Input: part model. Units: mm. Frame: model coordinates. A direction names the side the tool comes from. Coordinates: 2 decimals unless noted, no trailing zeros. Loops run counter-clockwise (first coordinate to the right, second up) from the corner with the lowest first, then second, coordinate; pieces in that order, holes last. Notation, with made-up numbers: (81, 26.25) - (93, 26.25) arc R18 cw to (93, 59.25) - close; hole circle Ø7 at (2, 59). An arc over 180 degrees is marked (long way). Use one line per item in the form item = value.
from build123d import *

# Parameters (mm, degrees)
F0_R     = 4.7
F0_R_2   = 1.5
F1_DEPTH = 7


with BuildPart() as f1:
    # F0 (on Top) → F1 (new body)
    with BuildSketch(Plane.XY):
        with BuildLine():
            Line((-26.979165, -28.984375), (-19.81169, -30.632258))
            ThreePointArc((-19.81169, -30.632258), (-8.174057, -35.553103), (4.444148, -36.208947))
            Line((4.444148, -36.208947), (11.611623, -37.85683))
            Line((11.611623, -37.85683), (16.622468, -32.473556))
            ThreePointArc((16.622468, -32.473556), (25.136294, -26.438703), (31.593175, -18.240328))
            ThreePointArc((31.593175, -18.240328), (32.647405, -16.278367), (33.579942, -14.255729))
            Line((33.579942, -14.255729), (38.590788, -8.872455))
            Line((38.590788, -8.872455), (36.434159, -1.841298))
            ThreePointArc((36.434159, -1.841298), (34.876919, 10.69761), (29.135794, 21.953219))
            Line((29.135794, 21.953219), (26.979165, 28.984375))
            Line((26.979165, 28.984375), (19.81169, 30.632258))
            ThreePointArc((19.81169, 30.632258), (10.328442, 34.988021), (0, 36.480657))
            ThreePointArc((0, 36.480657), (-2.226223, 36.412666), (-4.444148, 36.208947))
            Line((-4.444148, 36.208947), (-11.611623, 37.85683))
            Line((-11.611623, 37.85683), (-16.622468, 32.473556))
            ThreePointArc((-16.622468, 32.473556), (-26.702862, 24.855492), (-33.579942, 14.255729))
            Line((-33.579942, 14.255729), (-38.590788, 8.872455))
            Line((-38.590788, 8.872455), (-36.434159, 1.841298))
            ThreePointArc((-36.434159, 1.841298), (-35.464736, -8.549317), (-31.593175, -18.240328))
            ThreePointArc((-31.593175, -18.240328), (-30.421182, -20.134299), (-29.135794, -21.953219))
            Line((-29.135794, -21.953219), (-26.979165, -28.984375))
        make_face()
        with Locations((-14.546111, -25.194604)):
            Circle(F0_R, mode=Mode.SUBTRACT)
        with Locations((-25.194604, -14.546111)):
            Circle(F0_R, mode=Mode.SUBTRACT)
        with Locations((-29.092222, 0)):
            Circle(F0_R, mode=Mode.SUBTRACT)
        with Locations((-9.353936, -15.969821)):
            Circle(F0_R_2, mode=Mode.SUBTRACT)
        with BuildLine():
            Line((-6.784947, -19.181266), (-5.608941, -15.016094))
            ThreePointArc((-5.608941, -15.016094), (-0.212424, -16.028044), (5.209015, -15.159468))
            Line((5.209015, -15.159468), (6.635095, -19.233615))
            ThreePointArc((6.635095, -19.233615), (-0.079366, -20.345765), (-6.784947, -19.181266))
        make_face(mode=Mode.SUBTRACT)
        with BuildLine():
            Line((-20.003937, -3.714697), (-15.80879, -2.650562))
            ThreePointArc((-15.80879, -2.650562), (-13.986905, -7.830057), (-10.523976, -12.090874))
            Line((-10.523976, -12.090874), (-13.339252, -15.362969))
            ThreePointArc((-13.339252, -15.362969), (-17.659632, -10.104149), (-20.003937, -3.714697))
        make_face(mode=Mode.SUBTRACT)
        with Locations((0, -29.092222)):
            Circle(F0_R, mode=Mode.SUBTRACT)
        with Locations((14.546111, -25.194604)):
            Circle(F0_R, mode=Mode.SUBTRACT)
        with BuildLine():
            ThreePointArc((9.526279, -5.5), (0, -11), (-9.526279, -5.5))
            ThreePointArc((-9.526279, -5.5), (-9.526279, 5.5), (0, 11))
            ThreePointArc((0, 11), (9.526279, 5.5), (9.526279, -5.5))
        make_face(mode=Mode.SUBTRACT)
        with BuildLine():
            Line((13.21899, -15.466569), (10.199849, -12.365532))
            ThreePointArc((10.199849, -12.365532), (13.774481, -8.197987), (15.732992, -3.068594))
            Line((15.732992, -3.068594), (19.974347, -3.870647))
            ThreePointArc((19.974347, -3.870647), (17.580266, -10.241616), (13.21899, -15.466569))
        make_face(mode=Mode.SUBTRACT)
        with Locations((18.507238, -0.115835)):
            Circle(F0_R_2, mode=Mode.SUBTRACT)
        with Locations((25.194604, -14.546111)):
            Circle(F0_R, mode=Mode.SUBTRACT)
        with Locations((29.092222, 0)):
            Circle(F0_R, mode=Mode.SUBTRACT)
        with Locations((-25.194604, 14.546111)):
            Circle(F0_R, mode=Mode.SUBTRACT)
        with BuildLine():
            Line((-13.21899, 15.466569), (-10.199849, 12.365532))
            ThreePointArc((-10.199849, 12.365532), (-13.774481, 8.197987), (-15.732992, 3.068594))
            Line((-15.732992, 3.068594), (-19.974347, 3.870647))
            ThreePointArc((-19.974347, 3.870647), (-17.580266, 10.241616), (-13.21899, 15.466569))
        make_face(mode=Mode.SUBTRACT)
        with Locations((-9.153303, 16.085656)):
            Circle(F0_R_2, mode=Mode.SUBTRACT)
        with Locations((-14.546111, 25.194604)):
            Circle(F0_R, mode=Mode.SUBTRACT)
        with BuildLine():
            Line((20.003937, 3.714697), (15.80879, 2.650562))
            ThreePointArc((15.80879, 2.650562), (13.986905, 7.830057), (10.523976, 12.090874))
            Line((10.523976, 12.090874), (13.339252, 15.362969))
            ThreePointArc((13.339252, 15.362969), (17.659632, 10.104149), (20.003937, 3.714697))
        make_face(mode=Mode.SUBTRACT)
        with BuildLine():
            ThreePointArc((-6.635095, 19.233615), (0.079366, 20.345765), (6.784947, 19.181266))
            Line((6.784947, 19.181266), (5.608941, 15.016094))
            ThreePointArc((5.608941, 15.016094), (0.212424, 16.028044), (-5.209015, 15.159468))
            Line((-5.209015, 15.159468), (-6.635095, 19.233615))
        make_face(mode=Mode.SUBTRACT)
        with Locations((25.194604, 14.546111)):
            Circle(F0_R, mode=Mode.SUBTRACT)
        with Locations((14.546111, 25.194604)):
            Circle(F0_R, mode=Mode.SUBTRACT)
        with Locations((0, 29.092222)):
            Circle(F0_R, mode=Mode.SUBTRACT)
    extrude(amount=F1_DEPTH)


solid = f1.part
Q1. Cut plane A-A, the plane x = 23. Return loops of the section in (y, z).
Check values:
outline = (-28.32, 0) - (-18.7, 0) - (-18.7, 7) - (-28.32, 7) - close; (-10.39, 0) - (10.39, 0) - (10.39, 7) - (-10.39, 7) - close; (18.7, 0) - (29.9, 0) - (29.9, 7) - (18.7, 7) - close
Q2. First-contact query: P1, Ø3.5, axis at x = -9.15, y = 16.09, coming from the -Z side; P2, Ø1.5, axis at x = 16.5, z = 3.5, coming from the -Y side; P3, Ø2, axis at y = 30, z = 4.5, coming from the -X side; P4, Ø1.5, axis at x = -23, z = 1, coming from the +Y side. Flat tips, straight axial feed; report the tip coordinate or a pass-through.
Check values:
P1 = 0
P2 = -33.41
P3 = -22.13
P4 = 28.91
Q3. Cut plane B-B, the plane z = 3. Give the number of separate pieces and of enclosed holes in the cut face, then the cut area to 3 significant figures.
Check values:
separate_pieces = 1
enclosed_holes = 22
area = 2,740 mm²
Q4. Ray query, line 1 along X through (y, z) = (2.5, 3); line 2 along Y through (x, z) = (-5, 0.75); line 3 along Y through (x, z) = (3.5, 1). Return the intervals inside material, ascending. Write a range as [from, to].
Check values:
line_1 = [-36.64, -33.07], [-25.11, -10.71], [10.71, 25.11], [33.07, 36.39]
line_2 = [-36.14, -19.72], [-15.23, -9.8], [9.8, 15.23], [19.72, 36.34]
line_3 = [-36.31, -32.23], [-25.96, -20.04], [-15.64, -10.43], [10.43, 15.64], [20.04, 25.96], [32.23, 36.31]
Q5. Pull-direction query (X, two-part tool) for faces 1 (the flat face through (28.073, 25.42, 3.451)), 2 (the cylindrical face through (9.85, 25.4, 3.45)), 3 (the flat face through (8, 9, 7)); classes: pulls with the +X half, pulls with the -X half, needs draft (parallel to the pull), parting line crosses it, or undercut.
Check values:
face_1 = pulls with the +X half
face_2 = undercut
face_3 = needs draft
Q6. Set-up query: faces 4 (the cylindrical face through (25.03, -26.54, 3.45)), 5 (the cylindrical face through (14.024, 7.763, 3.451)). Return all of +Z, -Z, +X, -X, +Y, -Y with unobstructed straight access to the full face (end or side cutting, diameter ignored); none if empty.
Check values:
face_4 = +Z, -Z, +X, -Y
face_5 = +Z, -Z
